Source: CAD feature listing. Evaluate the final solid. Frame: model axes, mm. A direction names the side the tool comes from. Round coordinates to 2 decimals unless told otherwise and drop trailing zeros. Loops run counter-clockwise (first coordinate to the right, second up) from the corner with the lowest first, then second, coordinate; pieces in that order, holes last. Notation, with made-up numbers: (-4, -39) - (20, -39) arc R35 cw to (20, 0) - close; hole circle Ø10 at (10.5, 87.25). An arc over 180 degrees is marked (long way). One line per question, with ' | ' between items. Start each with the question number.
1. Cut plane B-B (x = 52). Return loops of the section in (y, z).
2. Ray query, line 1 (Z direction, x = 51.5, y = 29); line 2 (X direction, y = -24, z = 16); line 3 (Y direction, x = 56, z = 19). Return the intervals inside material, ascending.
3. Cut plane A-A (z = 16.5). Return loops of the section in (x, y).
4. Cut plane D-D (y = -13). Return loops of the section in (x, z), then the cut area to 3 significant figures.
5. Access query for faces 1 (the flat face through (20, -8, 12.7)), 2 (the flat face through (-1, 1, 0)). Directions: +Z, -Z, +X, -X, +Y, -Y. A direction counts if a zero-diameter tool reaches every point of the face in a straight line with its end or side. Return the directions, or none.
6. Mould query, pull axis X, two halves, no side actions, for faces 3 (the flat face through (48.146, -29.156, 25.222)), 4 (the flat face through (53, -33, 38.1)), 5 (the flat face through (60.671, -9, 10)). Classes: pulls with the +X half, pulls with the -X half, needs draft (parallel to the pull), parting line crosses it, or undercut.
7. Cut plane C-C (y = 8). Return loops of the section in (x, z), then the cut area to 3 significant figures.
```python
from build123d import *

# Parameters (mm, degrees)
F1_DEPTH = 12.7
F2_DEPTH = 38.1
F3_DEPTH = 38.1


with BuildPart() as f1:
    # F0 (on Top) → F1 (new body)
    with BuildSketch(Plane.XY):
        Polygon((60.671091, -19.528509), (60.671091, 39.057016), (-40.952984, -39.057016), (35.265073, -39.057016), align=None)
    extrude(amount=F1_DEPTH)

    # F0 (on Top) → F2 (join)
    with BuildSketch(Plane.XY):
        Polygon((60.671091, -39.057016), (60.671091, -19.528509), (35.265073, -39.057016), align=None)
    extrude(amount=F2_DEPTH)

    # F0 (on Top) → F3 (join)
    with BuildSketch(Plane.XY):
        Polygon((-40.952984, -39.057016), (60.671091, 39.057016), (-60.671091, 39.057016), (-60.671091, -39.057016), align=None)
    extrude(amount=F3_DEPTH)


solid = f1.part
```
Answers follow:
1) outline: (-39.06, 0) - (39.06, 0) - (39.06, 38.1) - (32.39, 38.1) - (32.39, 12.7) - (-26.19, 12.7) - (-26.19, 38.1) - (-39.06, 38.1) - close
2) line 1: z = 0 to 12.7 | line 2: x = -60.67 to -21.36, 54.85 to 60.67 | line 3: y = -39.06 to -23.12, 35.47 to 39.06
3) outline: (-60.67, -39.06) - (-40.95, -39.06) - (60.67, 39.06) - (-60.67, 39.06) - close; (35.27, -39.06) - (60.67, -39.06) - (60.67, -19.53) - close
4) outline: (-60.67, 0) - (60.67, 0) - (60.67, 12.7) - (-7.05, 12.7) - (-7.05, 38.1) - (-60.67, 38.1) - close | area: 2,900 mm2
5) face 1: +Z | face 2: -Z, +X, -X, +Y, -Y
6) face 3: undercut | face 4: needs draft | face 5: pulls with the +X half
7) outline: (-60.67, 0) - (60.67, 0) - (60.67, 12.7) - (20.27, 12.7) - (20.27, 38.1) - (-60.67, 38.1) - close | area: 3,600 mm2
